Source: three-view drawing plus pictorial views. Frame: mm from the lowest corner of the part. A direction names the side the tool comes from. Coordinates: 2 decimals unless noted, no trailing zeros. Order: outer loops, then holes, each group sorted by start corner. A loop starts at its lowest first (then second) coordinate and runs counter-clockwise, first axis right, second up. Notation, with made-up numbers: M -35,67.25 L -16,67.25 A12 ccw -16,87.25 Z; hole C -17.5,53.5 d3. An arc over 180 degrees is marked long. One line per question, with ' | ' between items.
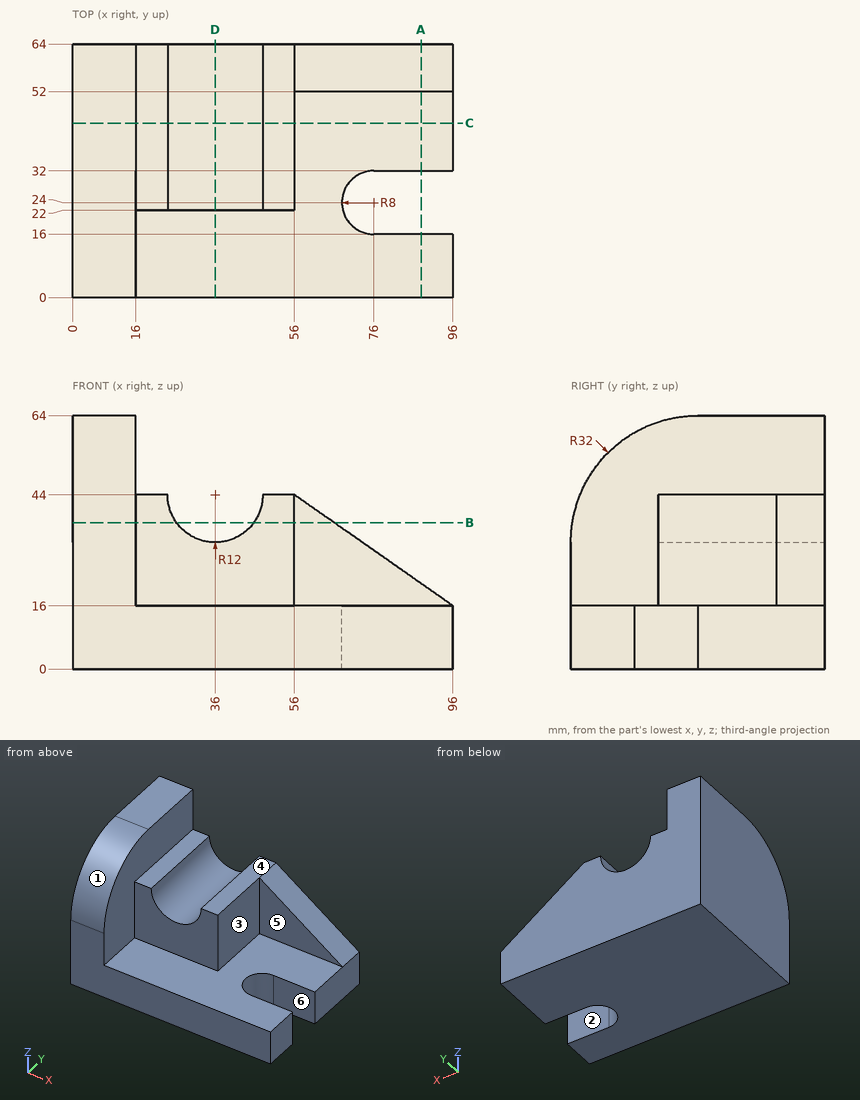
1. Pin query (flat end, axial travel): P1, Ø8.5, axis at x = 33, z = 26, coming from the -Y side; P2, Ø6, axis at y = 7.5, z = 50.5, coming from the +X side; P3, Ø2.5, axis at x = 21.5, y = 46.5, coming from the +Z side. Return the tip coordinate at first contact, or that it passes through.
Response values:
P1: stops at y = 22 | P2: stops at x = 16 | P3: stops at z = 44
2. Section D-D, the plane x = 36. Output: boundary loops of the cut face in (y, z).
Response values:
outline: M 0,0 L 64,0 L 64,32 L 22,32 L 22,16 L 0,16 Z
3. Section A-A, the plane x = 88. Output: boundary loops of the cut face in (y, z), and give its area (3 significant figures).
Response values:
outline: M 0,0 L 16,0 L 16,16 L 0,16 Z; M 32,0 L 64,0 L 64,21.6 L 52,21.6 L 52,16 L 32,16 Z | area: 835 mm^2
4. Section C-C, the plane y = 44. Output: boundary loops of the cut face in (x, z).
Response values:
outline: M 0,0 L 96,0 L 96,16 L 56,16 L 56,44 L 48,44 A12 cw 24,44 L 16,44 L 16,64 L 0,64 Z
5. Section B-B, the plane z = 37. Output: boundary loops of the cut face in (x, y), and give its area (3 significant figures).
Response values:
outline: M 0,0.39 L 16,0.39 L 16,22 L 26.25,22 L 26.25,64 L 0,64 Z; M 45.75,22 L 56,22 L 56,52 L 66,52 L 66,64 L 45.75,64 Z | area: 2,000 mm^2
6. Draft query along Y for the marked faces 1, 2 and 3. Return one class per face: pulls with the +Y half, pulls with the -Y half, needs draft (parallel to the pull), parting line crosses it, or undercut.
Response values:
face 1: pulls with the -Y half | face 2: undercut | face 3: needs draft
7. Material intervals for line 1 (X direction, y = 34, z = 50.5); line 2 (X direction, y = 38, z = 31), sorted ascending. Write a range as [from, to].
Response values:
line 1: x = [0, 16] | line 2: x = [0, 56]
8. Access query for the marked faces 4, 5 and 6. Directions: +Z, -Z, +X, -X, +Y, -Y. A direction counts if a zero-diameter tool reaches every point of the face in a straight line with its end or side. Return the directions, or none.
Response values:
face 4: +Z, +X, +Y, -Y | face 5: +Z, +X, -Y | face 6: +Z, -Z, +X
